```python
from build123d import *

# Parameters (mm, degrees)
BASE_EXTRUDE_DEPTH = 42.06875
SKETCH3_R          = 3.96875
CUT_EXTRUDE1_DEPTH = 85.842184608


with BuildPart() as part:
    # Sketch1 → Base-Extrude (new, symmetric)
    with BuildSketch(Plane.XY):
        Polygon((8.248891971, 0), (4.124445986, 7.14375), (-4.124445986, 7.14375), (-8.248891971, 0), (-4.124445986, -7.14375), (4.124445986, -7.14375), align=None)
    extrude(amount=BASE_EXTRUDE_DEPTH, both=True)

    # Sketch2 → Cut-Revolve1 (revolve, cut)
    with BuildSketch(Plane(origin=(0, 0, 0), x_dir=(0, 0, -1), z_dir=(1, 0, 0)), mode=Mode.PRIVATE) as cut_revolve1_sk:
        Polygon((19.84375, 6.35), (19.33575, 6.35), (19.33575, 8.89), (-19.33575, 8.89), (-19.33575, 6.35), (-19.84375, 6.35), (-19.84375, 8.89), (-31.600861032, 8.89), (-42.06875, 5.08), (-42.06875, 18.081978304), (42.06875, 18.081978304), (42.06875, 5.08), (31.600861032, 8.89), (19.84375, 8.89), align=None)
    revolve(cut_revolve1_sk.sketch.rotate(Axis((0, 0, 64.541972625), (0, 0, -1)), 90), axis=Axis((0, 0, 64.541972625), (0, 0, -1)), mode=Mode.SUBTRACT)

    # Sketch3 → Cut-Extrude1 (cut, through all)
    with BuildSketch(Plane.XY.offset(42.06875)):
        Circle(SKETCH3_R)
    extrude(amount=-CUT_EXTRUDE1_DEPTH, mode=Mode.SUBTRACT)


solid = part.part
```
For this review, take the finished solid that the model builds, in its own axes (mm). A direction names the side the tool comes from. Coordinates: 2 decimals unless noted, no trailing zeros. Order: outer loops, then holes, each group sorted by start corner. A loop starts at its lowest first (then second) coordinate and runs counter-clockwise, first axis right, second up. Notation, with made-up numbers: (81, 28.5) -> (127, 28.5) arc R28 ccw to (127, 64.5) -> close; hole circle Ø2 at (65.25, 40). An arc over 180 degrees is marked (long way). Answer as CSV lines item,"result".
Q1. We need section B-B (z = 23). State the section outline as (x, y) points.
Model answer:
outline,"(-8.25, 0) -> (-4.12, -7.14) -> (4.12, -7.14) -> (8.25, 0) -> (4.12, 7.14) -> (-4.12, 7.14) -> close; hole circle Ø7.94 at (0, 0)"
Q2. Clearance check with flat-ended pins moving along their axes: pin 1 Ø1 at (y, z) = (2, -15) entering from -X; pin 2 Ø6 at (y, z) = (-4, -30) entering from -X; pin 3 Ø1 at (y, z) = (-2, -27) entering from +X. State where each tip first meets the part, or that it passes through.
Model answer:
pin 1,"stops at x = -7.38"
pin 2,"stops at x = -7.67"
pin 3,"stops at x = 7.38"
Q3. For faces 1 (the face through (0, 7.144, -28)), 2 (the face through (-5.5, 3.7, -19.336)), list the 3-axis set-ups (+Z, -Z, +X, -X, +Y, -Y) from which the entire face can be reached by the end or side of a thin tool; tool diameter is ignored.
Model answer:
face 1,"+Z, -Z, +X, -X, +Y"
face 2,"none"
Q4. Wall thickness on line 1 along Y through (x, z) = (0, -11); line 2 along Z through (x, y) = (-3, 5.75); line 3 along Z through (x, y) = (5.5, -4.25): over which ranges is each line inside the solid? List them lowest first. Write a range as [from, to].
Model answer:
line 1,"y = [-7.14, -3.97], [3.97, 7.14]"
line 2,"z = [-38.21, -19.84], [-19.34, 19.34], [19.84, 38.21]"
line 3,"z = [-36.93, -19.84], [-19.34, 19.34], [19.84, 36.93]"
Q5. We need section A-A (x = 0). State the section outline as (y, z) points, plus the area to 3 significant figures.
Model answer:
outline,"(-7.14, -36.4) -> (-5.08, -42.07) -> (-3.97, -42.07) -> (-3.97, 42.07) -> (-5.08, 42.07) -> (-7.14, 36.4) -> (-7.14, 19.84) -> (-6.35, 19.84) -> (-6.35, 19.34) -> (-7.14, 19.34) -> (-7.14, -19.34) -> (-6.35, -19.34) -> (-6.35, -19.84) -> (-7.14, -19.84) -> close; (3.97, -42.07) -> (5.08, -42.07) -> (7.14, -36.4) -> (7.14, -19.84) -> (6.35, -19.84) -> (6.35, -19.34) -> (7.14, -19.34) -> (7.14, 19.34) -> (6.35, 19.34) -> (6.35, 19.84) -> (7.14, 19.84) -> (7.14, 36.4) -> (5.08, 42.07) -> (3.97, 42.07) -> close"
area,"509 mm2"
Q6. Draft analysis for pull direction Z (two halves, no side actions). For faces 3 (the face through (5.37, -1.69, -40.56)), 4 (the face through (-6.216, -3.522, -28.005)), 5 (the face through (-5.04, 3.86, 19.59)), state which applies: released by +Z, released by -Z, zero draft, split by the parting line, or undercut.
Model answer:
face 3,"released by -Z"
face 4,"zero draft"
face 5,"undercut"
